Verification items for this drawing (mm, ordinates from the low corner). A direction names the side the tool comes from. Give positions to 0.01 mm unless a question says otherwise; leave off trailing zeros. Loops run counter-clockwise (first coordinate to the right, second up) from the corner with the lowest first, then second, coordinate; pieces in that order, holes last. Notation, with made-up numbers: M 69,-23 L 126,-23 A34 ccw 126,12 Z; hole C 72,41.5 d11. An arc over 180 degrees is marked long. Answer in a Markdown table with one row per item.
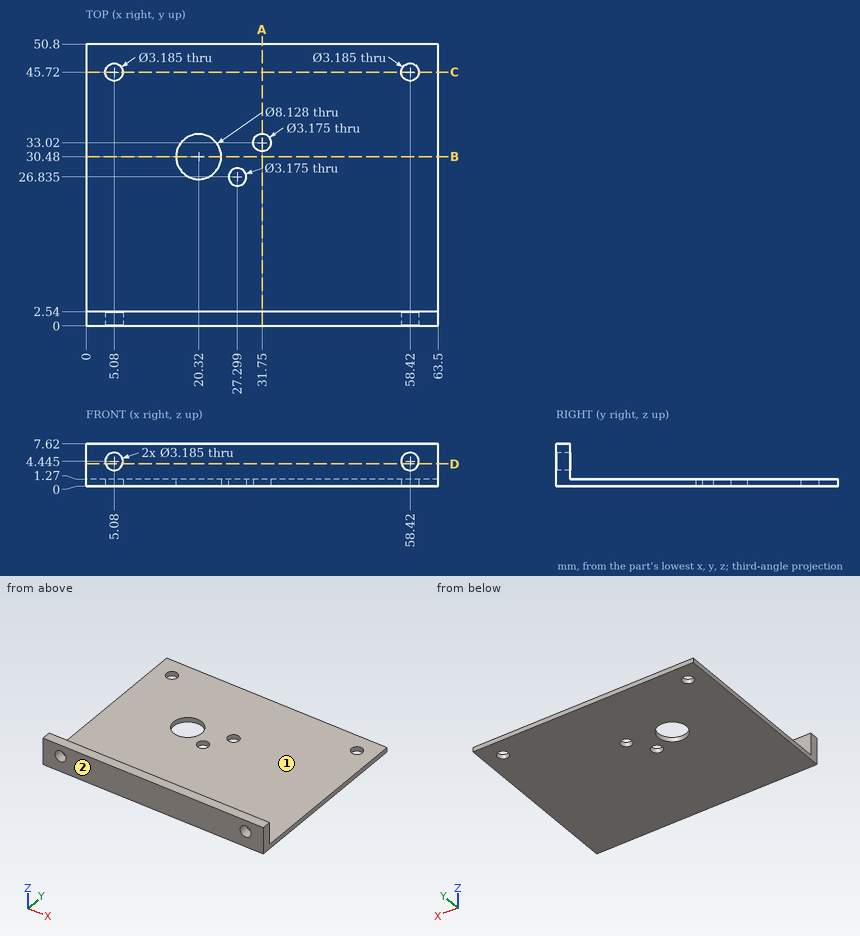
Item 1: Sectioned sample at B-B (y = 30.48). Record the cut outline in (x, z).
Reported:
| item | result |
|---|---|
| outline | M 0,0 L 16.26,0 L 16.26,1.27 L 0,1.27 Z; M 24.38,0 L 63.5,0 L 63.5,1.27 L 24.38,1.27 Z |
Item 2: Sectioned sample at D-D (z = 4). Record the cut outline in (x, y).
Reported:
| item | result |
|---|---|
| outline | M 0,0 L 3.55,0 L 3.55,2.54 L 0,2.54 Z; M 6.61,0 L 56.89,0 L 56.89,2.54 L 6.61,2.54 Z; M 59.95,0 L 63.5,0 L 63.5,2.54 L 59.95,2.54 Z |
Item 3: Tool access check on the marked faces 1 and 2. Record the directions out of +Z, -Z, +X, -X, +Y, -Y that give a thin tool (end or side, any length) a straight path to the whole face; none if there is none.
Reported:
| item | result |
|---|---|
| face 1 | +Z, +X, -X, +Y |
| face 2 | +Z, -Z, +X, -X, -Y |
Item 4: Scan lines: L1, parallel to X at y = 45.72, z = 0.4; L2, parallel to Y at x = 20.32, z = 0.5; L3, parallel to Z at x = 58.42, y = 1.95. Record each from-to range of solid material in increasing order. Write a range as [from, to].
Reported:
| item | result |
|---|---|
| L1 | x = [0, 3.49], [6.67, 56.83], [60.01, 63.5] |
| L2 | y = [0, 26.42], [34.54, 50.8] |
| L3 | z = [0, 2.85], [6.04, 7.62] |
Item 5: Sectioned sample at C-C (y = 45.72). Record the cut outline in (x, z).
Reported:
| item | result |
|---|---|
| outline | M 0,0 L 3.49,0 L 3.49,1.27 L 0,1.27 Z; M 6.67,0 L 56.83,0 L 56.83,1.27 L 6.67,1.27 Z; M 60.01,0 L 63.5,0 L 63.5,1.27 L 60.01,1.27 Z |
Item 6: Go/stop test with flat-tipped pins: pin 1 (2 mm diameter, centred on x = 30, y = 23.5, fed in from +Z); pin 2 (4 mm diameter, centred on x = 5.08, z = 4.445, fed in from +Y). Record where each tip stops, or that it passes through.
Reported:
| item | result |
|---|---|
| pin 1 | stops at z = 1.27 |
| pin 2 | stops at y = 2.54 |
Item 7: Sectioned sample at A-A (x = 31.75). Record the cut outline in (y, z).
Reported:
| item | result |
|---|---|
| outline | M 0,0 L 31.43,0 L 31.43,1.27 L 2.54,1.27 L 2.54,7.62 L 0,7.62 Z; M 34.61,0 L 50.8,0 L 50.8,1.27 L 34.61,1.27 Z |
